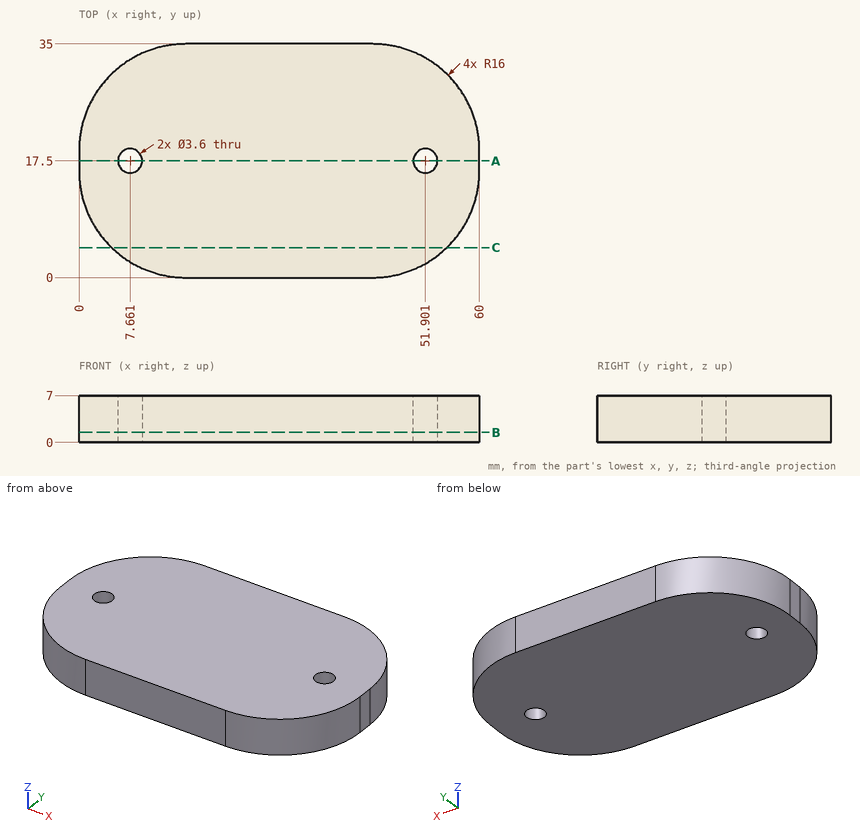
Geometry: see drawing. Coordinates: mm, zero at the bounding-box minimum. Give positions to 0.01 mm unless a question says otherwise; leave off trailing zeros. Write each loop counter-clockwise with the first axis right and the second up, starting at its lowest first coordinate (ties: lowest second). Pieces come first, ordered by that corner, then holes. Notation, with made-up numbers: M -8,88.25 L 41,88.25 A18 cw 41,107.25 Z; hole C 32,40.5 d4. An arc over 180 degrees is marked long. Return JSON: item names as keys, results as strings. Group by question number.
1) Ray query, L1, parallel to Y at x = 8, z = 2.5; L2, parallel to Y at x = 51, z = 1.75; L3, parallel to X at y = 20, z = 5.5. Return the intervals inside material, ascending.
2) Cut plane B-B, the plane z = 1.5. Output: boundary loops of the cut face in (x, y), then the cut area to 3 significant figures.
3) Cut plane C-C, the plane y = 4.5. Output: boundary loops of the cut face in (x, z).
4) Cut plane A-A, the plane y = 17.5. Output: boundary loops of the cut face in (x, z).
5) First-contact query: pin 1 Ø1.5 at (x, z) = (51.5, 5.5) entering from -Y; pin 2 Ø2 at (y, z) = (27, 3) entering from +X; pin 3 Ø4 at (x, z) = (12.5, 6) entering from -Y. Flat tips, straight axial feed; report the tip coordinate or a pass-through.
Data:
{
 "1": {"L1": "y = 2.14 to 15.73, 19.27 to 32.86", "L2": "y = 1.61 to 15.94, 19.06 to 33.39", "L3": "x = 0.03 to 59.97"},
 "2": {"outline": "M 0,16 A16 ccw 16,0 L 44,0 A16 ccw 60,16 L 60,19 A16 ccw 44,35 L 16,35 A16 ccw 0,19 Z; hole C 7.66,17.5 d3.6; hole C 51.9,17.5 d3.6", "area": "1,860 mm²"},
 "3": {"outline": "M 4.88,0 L 55.12,0 L 55.12,7 L 4.88,7 Z"},
 "4": {"outline": "M 0,0 L 5.86,0 L 5.86,7 L 0,7 Z; M 9.46,0 L 50.1,0 L 50.1,7 L 9.46,7 Z; M 53.7,0 L 60,0 L 60,7 L 53.7,7 Z"},
 "5": {"pin 1": "stops at y = 1.49", "pin 2": "stops at x = 58.39", "pin 3": "stops at y = 0.07"}
}
